```python
from build123d import *

# Parameters (mm, degrees)
F1_DEPTH = 2.5


with BuildPart() as f1:
    # F0 (on Front) → F1 (new body)
    with BuildSketch(Plane.XZ):
        with BuildLine():
            ThreePointArc((-38.431176, 54.871997), (-50.088537, 11.093074), (-9.038772, 30.260886))
            ThreePointArc((-9.038772, 30.260886), (-14.870959, 46.310651), (-29.646368, 54.871997))
            ThreePointArc((-29.646368, 54.871997), (-30.764385, 55.045527), (-31.889108, 55.168294))
            ThreePointArc((-31.889108, 55.168294), (-34.038772, 55.260886), (-36.188436, 55.168294))
            ThreePointArc((-36.188436, 55.168294), (-37.313159, 55.045527), (-38.431176, 54.871997))
        make_face()
        with BuildLine():
            ThreePointArc((-27.436737, 47.009275), (-26.647389, 46.676209), (-25.87478, 46.305967))
            ThreePointArc((-25.87478, 46.305967), (-24.07711, 45.256241), (-22.412639, 44.006009))
            Line((-22.412639, 44.006009), (-18.351048, 45.966118))
            ThreePointArc((-18.351048, 45.966118), (-17.663958, 46.033117), (-17.097186, 45.638972))
            Line((-17.097186, 45.638972), (-15.014567, 42.663804))
            ThreePointArc((-15.014567, 42.663804), (-14.840086, 41.978378), (-15.162712, 41.348962))
            Line((-15.162712, 41.348962), (-18.121272, 38.670913))
            ThreePointArc((-18.121272, 38.670913), (-16.90955, 35.800301), (-16.210955, 32.76375))
            Line((-16.210955, 32.76375), (-12.434427, 31.955754))
            ThreePointArc((-12.434427, 31.955754), (-11.866078, 31.606687), (-11.643643, 30.977885))
            Line((-11.643643, 30.977885), (-11.643643, 27.583928))
            ThreePointArc((-11.643643, 27.583928), (-11.910209, 26.904168), (-12.567791, 26.586809))
            Line((-12.567791, 26.586809), (-16.479693, 26.289224))
            ThreePointArc((-16.479693, 26.289224), (-17.186984, 23.927433), (-18.210327, 21.684425))
            Line((-18.210327, 21.684425), (-15.497295, 18.057033))
            ThreePointArc((-15.497295, 18.057033), (-15.301617, 17.374188), (-15.608727, 16.733679))
            Line((-15.608727, 16.733679), (-17.910432, 14.543347))
            ThreePointArc((-17.910432, 14.543347), (-18.514805, 14.271381), (-19.156508, 14.437057))
            Line((-19.156508, 14.437057), (-22.344594, 16.573609))
            ThreePointArc((-22.344594, 16.573609), (-22.868647, 16.142682), (-23.408566, 15.731809))
            ThreePointArc((-23.408566, 15.731809), (-25.41665, 14.457267), (-27.575226, 13.458566))
            Line((-27.575226, 13.458566), (-27.754484, 9.155613))
            ThreePointArc((-27.754484, 9.155613), (-28.038559, 8.498171), (-28.689408, 8.1993))
            Line((-28.689408, 8.1993), (-32.349118, 7.963827))
            ThreePointArc((-32.349118, 7.963827), (-33.001423, 8.152972), (-33.382452, 8.715194))
            Line((-33.382452, 8.715194), (-34.284313, 12.259912))
            ThreePointArc((-34.284313, 12.259912), (-37.014387, 12.505856), (-39.675475, 13.163432))
            Line((-39.675475, 13.163432), (-43.06656, 9.689531))
            ThreePointArc((-43.06656, 9.689531), (-43.698851, 9.391531), (-44.37184, 9.58043))
            Line((-44.37184, 9.58043), (-47.081775, 11.559113))
            ThreePointArc((-47.081775, 11.559113), (-47.457092, 12.104536), (-47.409397, 12.764896))
            Line((-47.409397, 12.764896), (-45.749935, 16.588138))
            ThreePointArc((-45.749935, 16.588138), (-47.841741, 18.70349), (-49.556617, 21.13445))
            Line((-49.556617, 21.13445), (-53.783735, 20.637289))
            ThreePointArc((-53.783735, 20.637289), (-54.451336, 20.795802), (-54.859614, 21.347279))
            Line((-54.859614, 21.347279), (-55.971582, 25.113494))
            ThreePointArc((-55.971582, 25.113494), (-55.918151, 25.820704), (-55.409183, 26.314619))
            Line((-55.409183, 26.314619), (-51.877978, 27.840539))
            ThreePointArc((-51.877978, 27.840539), (-51.97007, 28.659657), (-52.024569, 29.482132))
            ThreePointArc((-52.024569, 29.482132), (-51.977915, 31.771688), (-51.640984, 34.036798))
            Line((-51.640984, 34.036798), (-55.153296, 36.170466))
            ThreePointArc((-55.153296, 36.170466), (-55.58025, 36.701378), (-55.568044, 37.382559))
            Line((-55.568044, 37.382559), (-54.396808, 40.442881))
            ThreePointArc((-54.396808, 40.442881), (-53.971652, 40.946342), (-53.325566, 41.075976))
            Line((-53.325566, 41.075976), (-48.874356, 40.458966))
            ThreePointArc((-48.874356, 40.458966), (-47.087004, 42.664072), (-44.97527, 44.56083))
            Line((-44.97527, 44.56083), (-46.024426, 48.158616))
            ThreePointArc((-46.024426, 48.158616), (-45.98712, 48.824068), (-45.539929, 49.318274))
            Line((-45.539929, 49.318274), (-42.799457, 50.79961))
            ThreePointArc((-42.799457, 50.79961), (-42.125143, 50.899944), (-41.543224, 50.544788))
            Line((-41.543224, 50.544788), (-39.129262, 47.528842))
            ThreePointArc((-39.129262, 47.528842), (-36.360365, 48.113213), (-33.534103, 48.25646))
            Line((-33.534103, 48.25646), (-32.274634, 52.055594))
            ThreePointArc((-32.274634, 52.055594), (-31.828789, 52.605), (-31.130951, 52.721826))
            Line((-31.130951, 52.721826), (-27.811196, 52.06362))
            ThreePointArc((-27.811196, 52.06362), (-27.200088, 51.675185), (-27.01138, 50.976096))
            Line((-27.01138, 50.976096), (-27.436737, 47.009275))
        make_face(mode=Mode.SUBTRACT)
        with BuildLine():
            ThreePointArc((-31.889108, 55.168294), (-30.764385, 55.045527), (-29.646368, 54.871997))
            ThreePointArc((-29.646368, 54.871997), (-34.038772, 62.260886), (-38.431176, 54.871997))
            ThreePointArc((-38.431176, 54.871997), (-37.313159, 55.045527), (-36.188436, 55.168294))
            ThreePointArc((-36.188436, 55.168294), (-34.038772, 60.260886), (-31.889108, 55.168294))
        make_face()
        with BuildLine():
            ThreePointArc((-27.413909, 19.970899), (-23.295197, 24.400149), (-21.800608, 30.260886))
            ThreePointArc((-21.800608, 30.260886), (-23.053822, 35.655654), (-26.556799, 39.945551))
            ThreePointArc((-26.556799, 39.945551), (-27.302541, 40.478314), (-28.086061, 40.953775))
            ThreePointArc((-28.086061, 40.953775), (-39.463766, 41.230941), (-46.149733, 32.020793))
            ThreePointArc((-46.149733, 32.020793), (-46.245093, 31.143135), (-46.276935, 30.260886))
            ThreePointArc((-46.276935, 30.260886), (-40.524346, 19.882545), (-28.674625, 19.260951))
            ThreePointArc((-28.674625, 19.260951), (-28.033766, 19.597278), (-27.413909, 19.970899))
        make_face()
        with BuildLine():
            ThreePointArc((-26.494493, 36.076328), (-25.022157, 33.332721), (-24.513253, 30.260886))
            ThreePointArc((-24.513253, 30.260886), (-29.213352, 22.04804), (-38.675386, 21.939989))
            ThreePointArc((-38.675386, 21.939989), (-39.838521, 22.704536), (-40.877817, 23.630428))
            ThreePointArc((-40.877817, 23.630428), (-41.403861, 36.301662), (-28.874619, 38.265076))
            ThreePointArc((-28.874619, 38.265076), (-27.591004, 37.272434), (-26.494493, 36.076328))
        make_face(mode=Mode.SUBTRACT)
        with BuildLine():
            ThreePointArc((-46.276935, 30.260886), (-46.245093, 31.143135), (-46.149733, 32.020793))
            Line((-46.149733, 32.020793), (-52.024569, 29.482132))
            ThreePointArc((-52.024569, 29.482132), (-51.97007, 28.659657), (-51.877978, 27.840539))
            Line((-51.877978, 27.840539), (-46.276935, 30.260886))
        make_face()
        with BuildLine():
            Line((-22.344594, 16.573609), (-27.413909, 19.970899))
            ThreePointArc((-27.413909, 19.970899), (-28.033766, 19.597278), (-28.674625, 19.260951))
            Line((-28.674625, 19.260951), (-23.408566, 15.731809))
            ThreePointArc((-23.408566, 15.731809), (-22.868647, 16.142682), (-22.344594, 16.573609))
        make_face()
        with BuildLine():
            ThreePointArc((-28.086061, 40.953775), (-27.302541, 40.478314), (-26.556799, 39.945551))
            Line((-26.556799, 39.945551), (-25.87478, 46.305967))
            ThreePointArc((-25.87478, 46.305967), (-26.647389, 46.676209), (-27.436737, 47.009275))
            Line((-27.436737, 47.009275), (-28.086061, 40.953775))
        make_face()
        with BuildLine():
            Line((-36.404948, 32.222135), (-26.494493, 36.076328))
            ThreePointArc((-26.494493, 36.076328), (-27.591004, 37.272434), (-28.874619, 38.265076))
            Line((-28.874619, 38.265076), (-39.936242, 33.963191))
            ThreePointArc((-39.936242, 33.963191), (-40.489105, 33.433919), (-40.505786, 32.668734))
            Line((-40.505786, 32.668734), (-38.629208, 27.843408))
            ThreePointArc((-38.629208, 27.843408), (-38.099936, 27.290545), (-37.334751, 27.273864))
            Line((-37.334751, 27.273864), (-32.147718, 29.29111))
            ThreePointArc((-32.147718, 29.29111), (-31.382533, 29.274429), (-30.853261, 28.721566))
            Line((-30.853261, 28.721566), (-30.812855, 28.61767))
            ThreePointArc((-30.812855, 28.61767), (-30.829537, 27.852485), (-31.382399, 27.323213))
            Line((-31.382399, 27.323213), (-40.877817, 23.630428))
            ThreePointArc((-40.877817, 23.630428), (-39.838521, 22.704536), (-38.675386, 21.939989))
            Line((-38.675386, 21.939989), (-27.529152, 26.274779))
            ThreePointArc((-27.529152, 26.274779), (-26.976289, 26.804052), (-26.959608, 27.569237))
            Line((-26.959608, 27.569237), (-28.683195, 32.001171))
            ThreePointArc((-28.683195, 32.001171), (-29.212468, 32.554034), (-29.977653, 32.570715))
            Line((-29.977653, 32.570715), (-35.678317, 30.353717))
            ThreePointArc((-35.678317, 30.353717), (-36.443502, 30.370398), (-36.972774, 30.923261))
            Line((-36.972774, 30.923261), (-36.974492, 30.927678))
            ThreePointArc((-36.974492, 30.927678), (-36.957811, 31.692863), (-36.404948, 32.222135))
        make_face()
    extrude(amount=F1_DEPTH)


solid = f1.part
```
Work out the finished part from the listing and answer in its coordinate system (mm). Round coordinates to 2 decimals unless told otherwise and drop trailing zeros. Write each loop counter-clockwise with the first axis right and the second up, starting at its lowest first coordinate (ties: lowest second). Pieces come first, ordered by that corner, then holes. Notation, with made-up numbers: (7.25, 59.5) - (27.25, 59.5) arc R3 cw to (27.25, 63.5) - close; hole circle Ø6 at (33.25, 53.5). An arc over 180 degrees is marked (long way). Return JSON: item names as keys, results as strings. Group by question number.
Q1. Each of these flat-tipped pins is pushed along its axis until it touches: pin 1 Ø1 at (x, y) = (-25, -0.5) entering from -Z; pin 2 Ø3 at (x, z) = (-52.5, 39.5) entering from +Y; pin 3 Ø1 at (y, z) = (-0.5, 43.5) entering from -X. Where does it stop, or does it pass through?
Q2. Find the intervals of material crossed by L1, parallel to X at y = -0.45, z = 49.5; L2, parallel to Z at x = -49.5, y = -0.9; L3, parallel to Z at x = -50, y = -1.3 (3 decimals), in increasing order.
Q3. The part is cut by section C-C on z = 57.5. Write down the section's boundary in (x, y), then the cut area to 3 significant figures.
Q4. The part is cut by section D-D on y = -1.75. Count the separate pieces of the cut face and the enclosed holes in it, then the cut area to 3 significant figures.
Q5. The part is cut by section A-A on z = 10.5. Write down the section's boundary in (x, y).
Q6. The mould has two halves that part along Z. Classify faces 1 (the flat face through (-40.353, -1.232, 49.058)), 2 (the flat face through (-34, -2.5, 34)), 3 (the cylindrical face through (-31.84, -1.23, 52.6)): released by +Z, released by -Z, zero draft, split by the parting line, or undercut.
Q7. The part is cut by section B-B on x = -50.5. Write down the section's boundary in (y, z), then the cut area to 3 significant figures.
Solved:
{
 "1": {"pin 1": "z = 6.76", "pin 2": "y = 0", "pin 3": "x = -55.55"},
 "2": {"L1": "-50 to -45.2, -40.71 to -33.12, -27.17 to -18.07", "L2": "10.62 to 21.04, 28.87 to 30.57, 40.55 to 49.91", "L3": "11.019 to 21.082, 28.652 to 30.357, 40.615 to 49.502"},
 "3": {"outline": "(-39.03, -2.5) - (-37.03, -2.5) - (-37.03, 0) - (-39.03, 0) - close; (-31.05, -2.5) - (-29.04, -2.5) - (-29.04, 0) - (-31.05, 0) - close", "area": "10.0 mm²"},
 "4": {"separate pieces": "1", "enclosed holes": "6", "area": "1,060 mm²"},
 "5": {"outline": "(-49.35, -2.5) - (-45.63, -2.5) - (-45.63, 0) - (-49.35, 0) - close; (-42.28, -2.5) - (-33.84, -2.5) - (-33.84, 0) - (-42.28, 0) - close; (-27.7, -2.5) - (-18.73, -2.5) - (-18.73, 0) - (-27.7, 0) - close"},
 "6": {"face 1": "undercut", "face 2": "zero draft", "face 3": "undercut"},
 "7": {"outline": "(-2.5, 11.45) - (0, 11.45) - (0, 21.02) - (-2.5, 21.02) - close; (-2.5, 28.44) - (0, 28.44) - (0, 30.14) - (-2.5, 30.14) - close; (-2.5, 40.68) - (0, 40.68) - (0, 49.08) - (-2.5, 49.08) - close", "area": "49.2 mm²"}
}
